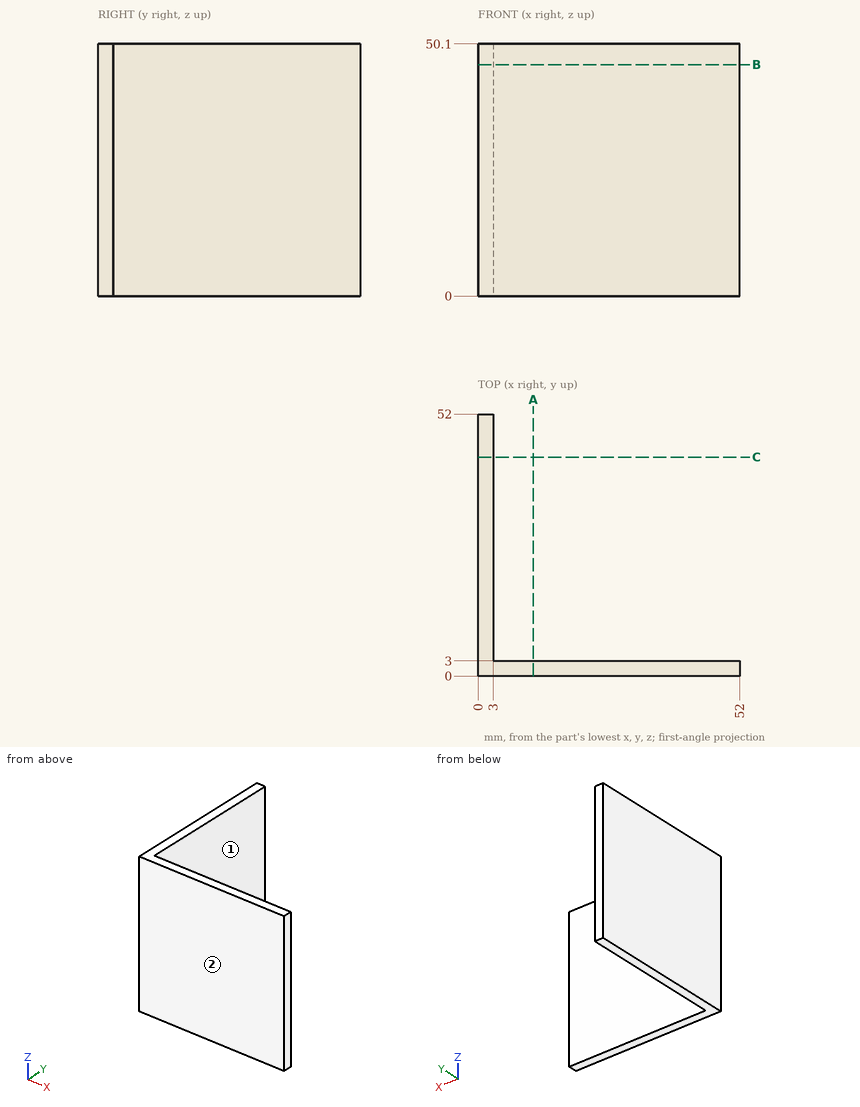
Here's the drawing with two shaded views (mm, measured from the low corner). I have some questions. A direction names the side the tool comes from. Coordinates: 2 decimals unless noted, no trailing zeros. Loops run counter-clockwise (first coordinate to the right, second up) from the corner with the lowest first, then second, coordinate; pieces in that order, holes last. Notation, with made-up numbers: (32.25, 31) - (62.25, 31) arc R18 ccw to (62.25, 50) - close; hole circle Ø8 at (37.5, 77.25). An arc over 180 degrees is marked (long way). Answer as CSV lines item,"result". Start each with the question number.
1) Which directions (+Z, -Z, +X, -X, +Y, -Y) give clear straight access to the entire face, cutting with the end or side of a thin tool? Please do the marked faces 1 and 2.
2) For pin 1 (8 mm diameter, centred on y = 40, z = 43, fed in from +X); pin 2 (24.5 mm diameter, centred on x = 16, z = 29.5, fed in from +Y), each with a flat end and sliding along its axis, tell me the tip position at first contact or that it passes through.
3) Suppose I cut it at A-A (x = 11). Please give me the cut outline in (y, z).
4) I need wall thicknesses on line 1 (Y direction, x = 20.5, z = 24.5). Which ranges of the line are inside material? Lowest first, please. Write a range as from..to.
5) Suppose I cut it at B-B (z = 46). Please give me the cut outline in (x, y).
Check result:
1,face 1,"+Z, -Z, +X, +Y"
1,face 2,"+Z, -Z, +X, -X, -Y"
2,pin 1,"stops at x = 3"
2,pin 2,"stops at y = 3"
3,outline,"(0, 0) - (3, 0) - (3, 50.1) - (0, 50.1) - close"
4,line 1,"y = 0..3"
5,outline,"(0, 0) - (52, 0) - (52, 3) - (3, 3) - (3, 52) - (0, 52) - close"
